Could you check a few things on this model? Use its own coordinates, in mm. Coordinates: 2 decimals unless noted, no trailing zeros. Write each loop counter-clockwise with the first axis right and the second up, starting at its lowest first coordinate (ties: lowest second). Pieces come first, ordered by that corner, then holes.
Item 1: If I drill on probe 1 along Y at (x, z) = (300, 10.75) (3 decimals); probe 2 along X at (y, z) = (266, 5.25), over which ranges is the centre line in solid material (lowest first)?
Item 2: For P1, Ø5, axis at x = 394, z = 8, coming from the -Y side, with a flat end and sliding along its axis, tell me the tip position at first contact or that it passes through.
Item 3: I want a section at C-C on z = 6. State how many separate pieces and enclosed holes the cut face has, then the cut area to 3 significant figures.
Item 4: I want a section at B-B on y = 350.5. Please give me the cut outline in (x, z).
Item 5: I want a section at A-A on x = 65.5. Please give me the cut outline in (y, z) (3 decimals), then the cut area to 3 significant figures.
Autodesk Inventor part; units mm, degrees
ref_plane "YZ Plane" through (0, 0, 0) normal (1, 0, 0) x (0, 1, 0)
ref_plane "XZ Plane" through (0, 0, 0) normal (0, 1, 0) x (-1, 0, 0)
ref_plane "XY Plane" through (0, 0, 0) normal (0, 0, 1) x (1, 0, 0)
sketch "Sketch1" plane through (0, 0, 0) normal (0, 0, 1) x (1, 0, 0)
  line L0 (0, 0) -> (457.2, 0)
  line L1 (457.2, 0) -> (457.2, 781.05)
  line L2 (457.2, 781.05) -> (0, 781.05)
  line L3 (0, 781.05) -> (0, 0)
  dimension "d0" = 457.2
  dimension "d1" = 781.05
extrude "Extrusion1" add sketch "Sketch1" along normal blind 19.05
sketch "Sketch2" plane through (0, 0, 19.05) normal (0, 0, 1) x (1, 0, 0)
  line L0 (0, 0) -> (457.2, 0)
  line L1 (457.2, 0) -> (457.2, 781.05)
  line L2 (457.2, 781.05) -> (0, 781.05)
  line L3 (0, 781.05) -> (0, 0)
  line L4 (25.4, 755.65) -> (220.6625, 755.65)
  line L5 (220.6625, 755.65) -> (220.6625, 403.225)
  line L6 (220.6625, 403.225) -> (25.4, 403.225)
  line L7 (25.4, 403.225) -> (25.4, 755.65)
  line L8 (246.0625, 755.65) -> (431.8, 755.65)
  line L9 (431.8, 755.65) -> (431.8, 403.225)
  line L10 (431.8, 403.225) -> (246.0625, 403.225)
  line L11 (246.0625, 403.225) -> (246.0625, 755.65)
  line L12 (25.4, 377.825) -> (220.6625, 377.825)
  line L13 (220.6625, 377.825) -> (220.6625, 25.4)
  line L14 (220.6625, 25.4) -> (25.4, 25.4)
  line L15 (25.4, 25.4) -> (25.4, 377.825)
  line L16 (246.0625, 377.825) -> (431.8, 377.825)
  line L17 (431.8, 377.825) -> (431.8, 25.4)
  line L18 (431.8, 25.4) -> (246.0625, 25.4)
  line L19 (246.0625, 25.4) -> (246.0625, 377.825)
  dimension "d24" = 25.4
  dimension "d25" = 25.4
  dimension "d26" = 25.4
  dimension "d27" = 25.4
  dimension "d28" = 25.4
  dimension "d29" = 25.4
  dimension "d30" = 25.4
  dimension "d31" = 25.4
  dimension "d32" = 25.4
  dimension "d33" = 25.4
  dimension "d34" = 185.7375
  dimension "d35" = 195.2625
  dimension "d36" = 352.425
extrude "Extrusion2" cut sketch "Sketch2" against normal blind 19.05 contours L4 L5 L6 L7 | L8 L9 L10 L11 | L12 L13 L14 L15 | L16 L17 L18 L19
properties part number "Door"
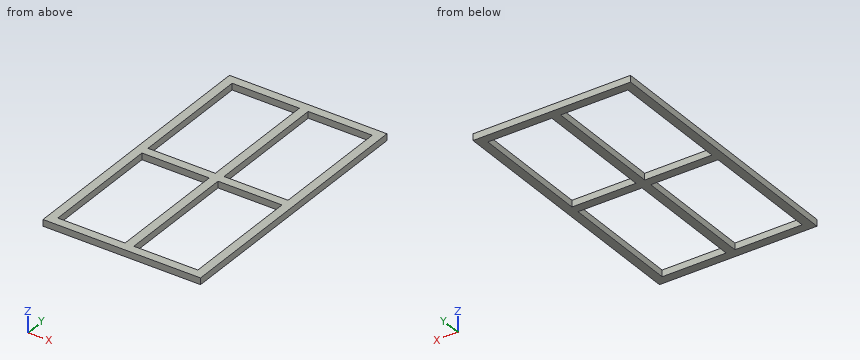
Response values:
1. probe 1: y = 0 to 25.4, 377.825 to 403.225, 755.65 to 781.05
1. probe 2: x = 0 to 25.4, 220.66 to 246.06, 431.8 to 457.2
2. P1: stops at y = 0
3. separate pieces: 1
3. enclosed holes: 4
3. area: 88,500 mm2
4. outline: (0, 0) - (25.4, 0) - (25.4, 19.05) - (0, 19.05) - close; (220.66, 0) - (246.06, 0) - (246.06, 19.05) - (220.66, 19.05) - close; (431.8, 0) - (457.2, 0) - (457.2, 19.05) - (431.8, 19.05) - close
5. outline: (0, 0) - (25.4, 0) - (25.4, 19.05) - (0, 19.05) - close; (377.825, 0) - (403.225, 0) - (403.225, 19.05) - (377.825, 19.05) - close; (755.65, 0) - (781.05, 0) - (781.05, 19.05) - (755.65, 19.05) - close
5. area: 1,450 mm2
